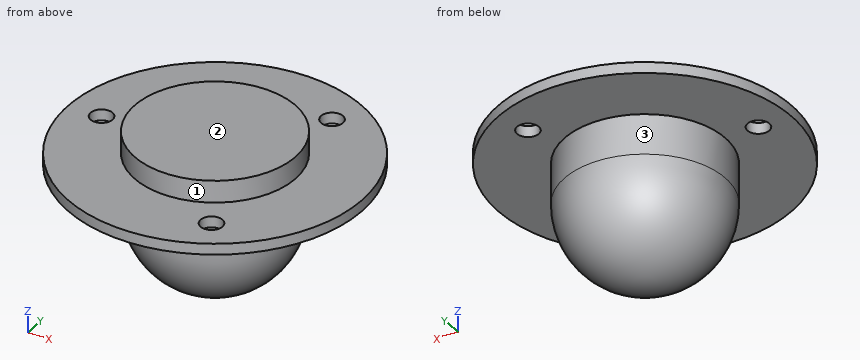
from build123d import *

# Parameters (mm, degrees)
SKETCH2_R                = 20.1
BOSS_EXTRUDE1_DEPTH      = 1.5
BOSS_EXTRUDE2_DEPTH      = 3
BOSS_EXTRUDE2_DEPTH_BACK = 18
SKETCH3_R                = 11
SKETCH4_R                = 1.5
CUT_EXTRUDE1_DEPTH       = 34.6455049
FILLET2_R                = 11


with BuildPart() as part:
    # Sketch2 → Boss-Extrude1 (new body)
    with BuildSketch(Plane.XY):
        Circle(SKETCH2_R)
    extrude(amount=BOSS_EXTRUDE1_DEPTH)

    # Sketch3 → Boss-Extrude2 (add, two sides: drawn at the far end of the back side and taken through both)
    with BuildSketch(Plane.XY.offset(1.5).offset(-BOSS_EXTRUDE2_DEPTH_BACK)):
        Circle(SKETCH3_R)
    extrude(amount=BOSS_EXTRUDE2_DEPTH + BOSS_EXTRUDE2_DEPTH_BACK)

    # Sketch4 → Cut-Extrude1 (cut, through all)
    with BuildSketch(Plane.XY.offset(1.5)):
        with Locations((-15.55, 0)):
            Circle(SKETCH4_R)
        with Locations((7.775, 13.466695029)):
            Circle(SKETCH4_R)
        with Locations((7.775, -13.466695029)):
            Circle(SKETCH4_R)
    extrude(amount=-CUT_EXTRUDE1_DEPTH, mode=Mode.SUBTRACT)

    # Fillet2
    fillet2_edges = [part.edges().sort_by_distance(p)[0] for p in [
        (-11, 0, -16.5),
    ]]
    fillet(fillet2_edges, radius=FILLET2_R)


solid = part.part
Could you check a few things on this model? Use its own coordinates, in mm. Face numbers are marked on the shaded views. A direction names the side the tool comes from. Coordinates: 2 decimals unless noted, no trailing zeros. Order: outer loops, then holes, each group sorted by start corner. A loop starts at its lowest first (then second) coordinate and runs counter-clockwise, first axis right, second up. Notation, with made-up numbers: (75.5, 61.25) -> (130.5, 61.25) arc R30 cw to (130.5, 98.25) -> close; hole circle Ø8 at (29.5, 59). An arc over 180 degrees is marked (long way). One line per item, written item: value. Start each with the question number.
1) If I drill on L1, parallel to Y at x = 0.5, z = -2; L2, parallel to Z at x = 6, y = 12; L3, parallel to Z at x = 7, y = 5.5, over which ranges is the centre line in solid material (lowest first)? Write a range as [from, to].
2) Imagine slicing it at D-D on z = 2.75. List the corners of the cut face in (x, y) for me.
3) Which directions (+Z, -Z, +X, -X, +Y, -Y) give clear straight access to the entire face, cutting with the end or side of a thin tool? Please do the marked faces 1, 2 and 3.
4) Imagine slicing it at A-A on y = 0. List the corners of the cut face in (x, z) for me.
5) I'm going to push flat-ended pins straight in: pin 1 (3.5 mm diameter, centred on x = 7.78, y = 13.47, fed in from -Z); pin 2 (12 mm diameter, centred on x = -14.5, z = -8.5, fed in from -Y); pin 3 (2 mm diameter, centred on y = -4, z = -8, fed in from -X); pin 4 (2.5 mm diameter, centred on x = -15.55, y = 0, fed in from -Z). Where does each tip first touch, or does it pass through?
6) Imagine slicing it at C-C on x = 0. List the corners of the cut face in (y, z) for me, plus the area to 3 significant figures.
7) Imagine slicing it at B-B on x = -15.55. List the corners of the cut face in (y, z) for me.
Answer list:
1. L1: y = [-10.99, 10.99]
1. L2: z = [0, 1.5]
1. L3: z = [-11.96, 4.5]
2. outline: circle Ø22 at (0, 0)
3. face 1: +Z
3. face 2: +Z, +X, -X, +Y, -Y
3. face 3: -Z
4. outline: (-20.1, 0) -> (-17.05, 0) -> (-17.05, 1.5) -> (-20.1, 1.5) -> close; (-14.05, 0) -> (-11, 0) -> (-11, -5.5) arc R11 ccw to (11, -5.5) -> (11, 0) -> (20.1, 0) -> (20.1, 1.5) -> (11, 1.5) -> (11, 4.5) -> (-11, 4.5) -> (-11, 1.5) -> (-14.05, 1.5) -> close
5. pin 1: stops at z = 0
5. pin 2: stops at y = -6.59
5. pin 3: stops at x = -10.35
5. pin 4: passes through
6. outline: (-20.1, 0) -> (-11, 0) -> (-11, -5.5) arc R11 ccw to (11, -5.5) -> (11, 0) -> (20.1, 0) -> (20.1, 1.5) -> (11, 1.5) -> (11, 4.5) -> (-11, 4.5) -> (-11, 1.5) -> (-20.1, 1.5) -> close
6. area: 437 mm2
7. outline: (-12.74, 0) -> (-1.5, 0) -> (-1.5, 1.5) -> (-12.74, 1.5) -> close; (1.5, 0) -> (12.74, 0) -> (12.74, 1.5) -> (1.5, 1.5) -> close
